from build123d import *

# Parameters (mm, degrees)
ESQUISSE1_W             = 13
ESQUISSE1_H             = 0.5
BOSS_EXTRU_1_DEPTH      = 220
ENL_V_MAT_EXTRU_1_REACH = 222.384
ESQUISSE2_R             = 2


with BuildPart() as part:
    # Esquisse1 → Boss.-Extru.1 (new body)
    with BuildSketch(Plane.XY):
        with Locations((6.5, 0.25)):
            Rectangle(ESQUISSE1_W, ESQUISSE1_H)
    extrude(amount=BOSS_EXTRU_1_DEPTH)

    # Esquisse2 → Enlèv. mat.-Extru.1 (cut, up to next)
    with BuildSketch(Plane(origin=(0, 0.5, 0), x_dir=(1, 0, 0), z_dir=(0, 1, 0)), mode=Mode.PRIVATE) as enl_v_mat_extru_1_sk1:
        with Locations(Location((5, -45, 0), (0, 0, 270))):
            Circle(ESQUISSE2_R)
    enl_v_mat_extru_1_tool1 = extrude(enl_v_mat_extru_1_sk1.sketch, amount=-ENL_V_MAT_EXTRU_1_REACH, mode=Mode.PRIVATE) & part.part
    # Esquisse2 → Enlèv. mat.-Extru.1 (cut, up to next)
    with BuildSketch(Plane(origin=(0, 0.5, 0), x_dir=(1, 0, 0), z_dir=(0, 1, 0)), mode=Mode.PRIVATE) as enl_v_mat_extru_1_sk2:
        with Locations(Location((5, -105, 0), (0, 0, 270))):
            Circle(ESQUISSE2_R)
    enl_v_mat_extru_1_tool2 = extrude(enl_v_mat_extru_1_sk2.sketch, amount=-ENL_V_MAT_EXTRU_1_REACH, mode=Mode.PRIVATE) & part.part
    # Esquisse2 → Enlèv. mat.-Extru.1 (cut, up to next)
    with BuildSketch(Plane(origin=(0, 0.5, 0), x_dir=(1, 0, 0), z_dir=(0, 1, 0)), mode=Mode.PRIVATE) as enl_v_mat_extru_1_sk3:
        with Locations(Location((5, -165, 0), (0, 0, 270))):
            Circle(ESQUISSE2_R)
    enl_v_mat_extru_1_tool3 = extrude(enl_v_mat_extru_1_sk3.sketch, amount=-ENL_V_MAT_EXTRU_1_REACH, mode=Mode.PRIVATE) & part.part
    add(enl_v_mat_extru_1_tool1.solids().sort_by_distance((5, 0.5, 45))[0], mode=Mode.SUBTRACT)
    add(enl_v_mat_extru_1_tool2.solids().sort_by_distance((5, 0.5, 105))[0], mode=Mode.SUBTRACT)
    add(enl_v_mat_extru_1_tool3.solids().sort_by_distance((5, 0.5, 165))[0], mode=Mode.SUBTRACT)


solid = part.part
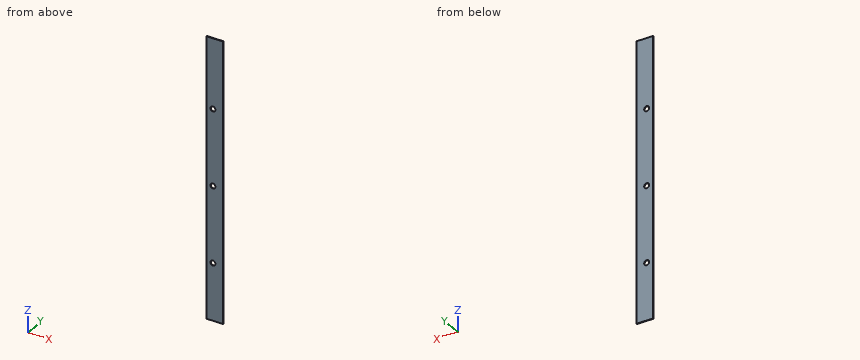
Model file for the job. Use its own axes, mm. Round coordinates to 2 decimals unless told otherwise and drop trailing zeros. Loops run counter-clockwise (first coordinate to the right, second up) from the corner with the lowest first, then second, coordinate; pieces in that order, holes last.
1. Drop flat-ended pins along their axis: P1, Ø3, axis at x = 5, z = 45, coming from the -Y side; P2, Ø4.5, axis at x = 5, z = 165, coming from the -Y side. Give the stop position or say it passes through.
Check values:
P1: passes through
P2: stops at y = 0
2. Band-saw the part on A-A, the plane z = 165. List the corners of the cut face in (x, y), and give its area (3 significant figures).
Check values:
outline: (0, 0) - (3, 0) - (3, 0.5) - (0, 0.5) - close; (7, 0) - (13, 0) - (13, 0.5) - (7, 0.5) - close
area: 4.50 mm2
3. Band-saw the part on B-B, the plane x = 5. List the corners of the cut face in (y, z), and give its area (3 significant figures).
Check values:
outline: (0, 0) - (0.5, 0) - (0.5, 43) - (0, 43) - close; (0, 47) - (0.5, 47) - (0.5, 103) - (0, 103) - close; (0, 107) - (0.5, 107) - (0.5, 163) - (0, 163) - close; (0, 167) - (0.5, 167) - (0.5, 220) - (0, 220) - close
area: 104 mm2
4. Wall check: probe 1 along X at (y, z) = (0.2, 105); probe 2 along Z at (x, y) = (4.75, 0.15); probe 3 along Z at (x, y) = (3.25, 0.35). Give the ranges that are in metal, low to high.
Check values:
probe 1: x = 0 to 3, 7 to 13
probe 2: z = 0 to 43.02, 46.98 to 103.02, 106.98 to 163.02, 166.98 to 220
probe 3: z = 0 to 44.03, 45.97 to 104.03, 105.97 to 164.03, 165.97 to 220
